```python
from build123d import *

# Parameters (mm, degrees)
CROQUIS1_R              = 8
CROQUIS1_R_2            = 1.55
SALIENTE_EXTRUIR1_DEPTH = 3.5
CROQUIS2_R              = 1.55
CORTAR_EXTRUIR1_DEPTH   = 157.957648109
CROQUIS3_R              = 5
CORTAR_EXTRUIR2_DEPTH   = 10


with BuildPart() as part:
    # Croquis1 → Saliente-Extruir1 (new body)
    with BuildSketch(Plane(origin=(0, 0, 0), x_dir=(1, 0, 0), z_dir=(0, 1, 0))):
        with BuildLine():
            Line((-75.83, 106.96), (-75.83, 36.96))
            Line((-75.83, 36.96), (-69.88, 31.76))
            Line((-69.88, 31.76), (-69.88, -51.39))
            Line((-69.88, -51.39), (-75.83, -56.59))
            Line((-75.83, -56.59), (-75.83, -112.67))
            ThreePointArc((-75.83, -112.67), (-72.813199846, -119.953199846), (-65.53, -122.97))
            ThreePointArc((-65.53, -122.97), (-51.316231926, -121.339014909), (-37.841336827, -116.530842982))
            ThreePointArc((-37.841336827, -116.530842982), (0, -107.730623626), (37.841336827, -116.530842982))
            ThreePointArc((37.841336827, -116.530842982), (51.316231926, -121.339014909), (65.53, -122.97))
            ThreePointArc((65.53, -122.97), (72.813199846, -119.953199846), (75.83, -112.67))
            Line((75.83, -112.67), (75.83, -56.59))
            Line((75.83, -56.59), (69.88, -51.39))
            Line((69.88, -51.39), (69.88, 31.76))
            Line((69.88, 31.76), (75.83, 36.96))
            Line((75.83, 36.96), (75.83, 106.96))
            ThreePointArc((75.83, 106.96), (0, 137.38), (-75.83, 106.96))
        make_face()
        with Locations(Location((0, 32.92, 0), (0, 0, 270))):
            Circle(CROQUIS1_R, mode=Mode.SUBTRACT)
        with Locations(Location((69.23, -114.59, 0), (0, 0, 270))):
            Circle(CROQUIS1_R_2, mode=Mode.SUBTRACT)
        with Locations(Location((0, -32.92, 0), (0, 0, 90))):
            Circle(CROQUIS1_R, mode=Mode.SUBTRACT)
        with Locations(Location((-69.23, -114.59, 0), (0, 0, 90))):
            Circle(CROQUIS1_R_2, mode=Mode.SUBTRACT)
        with BuildLine():
            Line((-7.895, -88.57), (7.895, -88.57))
            ThreePointArc((7.895, -88.57), (13.91, -82.555), (7.895, -76.54))
            Line((7.895, -76.54), (-7.895, -76.54))
            ThreePointArc((-7.895, -76.54), (-13.91, -82.555), (-7.895, -88.57))
        make_face(mode=Mode.SUBTRACT)
        with BuildLine():
            Line((-7.895, 88.57), (7.895, 88.57))
            ThreePointArc((7.895, 88.57), (13.91, 82.555), (7.895, 76.54))
            Line((7.895, 76.54), (-7.895, 76.54))
            ThreePointArc((-7.895, 76.54), (-13.91, 82.555), (-7.895, 88.57))
        make_face(mode=Mode.SUBTRACT)
        with BuildLine():
            Line((-13.415, 120.93), (13.415, 120.93))
            ThreePointArc((13.415, 120.93), (14.915, 119.43), (13.415, 117.93))
            Line((13.415, 117.93), (-13.415, 117.93))
            ThreePointArc((-13.415, 117.93), (-14.915, 119.43), (-13.415, 120.93))
        make_face(mode=Mode.SUBTRACT)
    extrude(amount=SALIENTE_EXTRUIR1_DEPTH)

    # Croquis2 → Cortar-Extruir1 (cut, through all)
    with BuildSketch(Plane(origin=(0, 3.5, 0), x_dir=(1, 0, 0), z_dir=(0, 1, 0))):
        with Locations(Location((-60.88, 66.51, 0), (0, 0, 270))):
            Circle(CROQUIS2_R)
        with Locations(Location((-60.88, 96.51, 0), (0, 0, 270))):
            Circle(CROQUIS2_R)
        with Locations(Location((-36.88, 96.51, 0), (0, 0, 270))):
            Circle(CROQUIS2_R)
        with Locations(Location((-36.88, 66.51, 0), (0, 0, 270))):
            Circle(CROQUIS2_R)
        with Locations(Location((60.88, 66.51, 0), (0, 0, 90))):
            Circle(CROQUIS2_R)
        with Locations(Location((36.88, 66.51, 0), (0, 0, 90))):
            Circle(CROQUIS2_R)
        with Locations(Location((36.88, 96.51, 0), (0, 0, 90))):
            Circle(CROQUIS2_R)
        with Locations(Location((60.88, 96.51, 0), (0, 0, 90))):
            Circle(CROQUIS2_R)
        with Locations(Location((60.88, -96.51, 0), (0, 0, 270))):
            Circle(CROQUIS2_R)
        with Locations(Location((36.88, -96.51, 0), (0, 0, 270))):
            Circle(CROQUIS2_R)
        with Locations(Location((36.88, -66.51, 0), (0, 0, 270))):
            Circle(CROQUIS2_R)
        with Locations(Location((60.88, -66.51, 0), (0, 0, 270))):
            Circle(CROQUIS2_R)
        with Locations(Location((-36.88, -66.51, 0), (0, 0, 90))):
            Circle(CROQUIS2_R)
        with Locations(Location((-36.88, -96.51, 0), (0, 0, 90))):
            Circle(CROQUIS2_R)
        with Locations(Location((-60.88, -96.51, 0), (0, 0, 90))):
            Circle(CROQUIS2_R)
        with Locations(Location((-60.88, -66.51, 0), (0, 0, 90))):
            Circle(CROQUIS2_R)
    extrude(amount=-CORTAR_EXTRUIR1_DEPTH, mode=Mode.SUBTRACT)

    # Croquis3 → Cortar-Extruir2 (cut)
    with BuildSketch(Plane(origin=(0, 3.5, 0), x_dir=(1, 0, 0), z_dir=(0, 1, 0))):
        with Locations(Location((0, 0, 0), (0, 0, 270))):
            Circle(CROQUIS3_R)
    extrude(amount=-CORTAR_EXTRUIR2_DEPTH, mode=Mode.SUBTRACT)


solid = part.part
```
Part model, mm, in its own coordinate system. A direction names the side the tool comes from. Coordinates: 2 decimals unless noted, no trailing zeros. Loops run counter-clockwise (first coordinate to the right, second up) from the corner with the lowest first, then second, coordinate; pieces in that order, holes last. Notation, with made-up numbers: (-7, 16) - (15, 16) arc R19 ccw to (15, 32) - close; hole circle Ø10 at (-21.5, 47). An arc over 180 degrees is marked (long way). Write item = value, one per line. Start each with the question number.
Item 1: Mould opens along Z. For faces 4 (the cylindrical face through (-13.91, 1.73, -82.42)), 5 (the cylindrical face through (-72.893, 1.726, 119.873)), 6 (the flat face through (-1, 3.5, -9)) say: released by +Z, released by -Z, zero draft, split by the parting line, or undercut.
Item 2: Cut at D-D, the plane z = 85.5. Give the cut face in (x, y), and give its area (3 significant figures).
Item 3: 3-axis set-ups, long thin cutter, end or side, ignore diameter. For faces 1 (the flat face through (-72.81, 1.73, 53.95)), 2 (the flat face through (72.9, 1.73, 54.03)), 3 (the cylindrical face through (51.121, 1.726, 121.293)): which of +Z, -Z, +X, -X, +Y, -Y reach the whole face in a straight line?
Item 4: Cut at A-A, the plane z = 0. Give the cut face in (x, y).
Item 5: Wall check: L1, parallel to X at y = 1.85, z = 0; L2, parallel to Z at x = 7, y = 0.9; L3, parallel to X at y = 2.85, z = -96. Give the ranges that are in metal, low to high. Write a range as from..to.
Item 6: Cut at B-B, the plane x = 0. Give the cut face in (y, z).
Item 7: Cut at C-C, the plane y = 1.25. State how many separate pieces and enclosed holes the cut face has, and give its area (3 significant figures).
Item 8: Flat gauge pins, fed straight in: pin 1 Ø11.5 at (x, z) = (0, 0) entering from -Y; pin 2 Ø1.8 at (y, z) = (2, 5.5) entering from -X; pin 3 Ø3 at (x, z) = (60.88, 66.51) entering from -Y; pin 4 Ø1.5 at (x, y) = (45.5, 1) entering from -Z. Where does each tip first touch, or does it go through?
The answers:
q1.face_4 = undercut
q1.face_5 = released by +Z
q1.face_6 = zero draft
q2.outline = (-75.83, 0) - (-13.14, 0) - (-13.14, 3.5) - (-75.83, 3.5) - close; (13.14, 0) - (75.83, 0) - (75.83, 3.5) - (13.14, 3.5) - close
q2.area = 439 mm2
q3.face_1 = -X, +Y, -Y
q3.face_2 = +X, +Y, -Y
q3.face_3 = +Z, +Y, -Y
q4.outline = (-69.88, 0) - (-5, 0) - (-5, 3.5) - (-69.88, 3.5) - close; (5, 0) - (69.88, 0) - (69.88, 3.5) - (5, 3.5) - close
q5.L1 = -69.88..-5, 5..69.88
q5.L2 = -137.16..-120.93, -117.93..-88.57, -76.54..-36.79, -29.05..29.05, 36.79..76.54, 88.57..108.02
q5.L3 = -75.83..-62.34, -59.42..-38.34, -35.42..35.42, 38.34..59.42, 62.34..75.83
q6.outline = (0, -137.38) - (3.5, -137.38) - (3.5, -120.93) - (0, -120.93) - close; (0, -117.93) - (3.5, -117.93) - (3.5, -88.57) - (0, -88.57) - close; (0, -76.54) - (3.5, -76.54) - (3.5, -40.92) - (0, -40.92) - close; (0, -24.92) - (3.5, -24.92) - (3.5, -5) - (0, -5) - close; (0, 5) - (3.5, 5) - (3.5, 24.92) - (0, 24.92) - close; (0, 40.92) - (3.5, 40.92) - (3.5, 76.54) - (0, 76.54) - close; (0, 88.57) - (3.5, 88.57) - (3.5, 107.73) - (0, 107.73) - close
q7.separate_pieces = 1
q7.enclosed_holes = 24
q7.area = 34,600 mm2
q8.pin_1 = 0
q8.pin_2 = -69.88
q8.pin_3 = through
q8.pin_4 = -127.84
